The listing builds one solid part. Answer for the finished solid, in the listing's coordinates (mm). Round coordinates to 2 decimals unless told otherwise and drop trailing zeros. Loops run counter-clockwise (first coordinate to the right, second up) from the corner with the lowest first, then second, coordinate; pieces in that order, holes last. Notation, with made-up numbers: (-35, -36.5) -> (-28, -36.5) arc R23 ccw to (-28, 2.5) -> close; hole circle Ø4 at (28, -10). An arc over 180 degrees is marked (long way). One line per question, with ' | ' between items.
from build123d import *

# Parameters (mm, degrees)
SKETCH1_W           = 75
SKETCH1_H           = 60
BOSS_EXTRUDE1_DEPTH = 70
CAVITY1_START       = 5
CAVITY1_OUTLINE_R   = 0.75
CAVITY1_DEPTH       = 55.9
CAVITY1_2_OUTLINE_R = 0.75
CAVITY1_2_DEPTH     = 31.4
CAVITY1_START_2     = 13
CAVITY1_3_OUTLINE_R = 0.75
CAVITY1_3_DEPTH     = 47.9
CAVITY1_4_OUTLINE_R = 0.75
CAVITY1_4_DEPTH     = 23.4


# Read off the part's stored shape, not the designer's step: Cavity1
with BuildPart() as part:
    # Sketch1 → Boss-Extrude1 (new body)
    with BuildSketch(Plane.XY):
        with Locations((37.5, 30)):
            Rectangle(SKETCH1_W, SKETCH1_H)
    extrude(amount=BOSS_EXTRUDE1_DEPTH)

    # Cavity1 outline → Cavity1 (cut)
    with BuildSketch(Plane.XY.offset(CAVITY1_START)):
        with BuildLine():
            Line((18.46548662, 52.336946082), (7.908006381, 37.670492946))
            Line((7.908006381, 37.670492946), (9.936997433, 36.209946709))
            ThreePointArc((9.936997433, 36.209946709), (8.94403376, 33.444468797), (9.567109894, 30.572949848))
            Line((9.567109894, 30.572949848), (8.245641386, 29.863216812))
            Line((8.245641386, 29.863216812), (18.37116603, 11.010266096))
            Line((18.37116603, 11.010266096), (21.895082052, 12.902887525))
            Line((21.895082052, 12.902887525), (11.769557408, 31.755838241))
            ThreePointArc((11.769557408, 31.755838241), (11.438668953, 33.280776232), (11.965988485, 34.749400472))
            Line((11.965988485, 34.749400472), (20.056953769, 45.989370661))
            ThreePointArc((20.056953769, 45.989370661), (21.356620935, 46.794592998), (22.845349854, 46.446449406))
            ThreePointArc((22.845349854, 46.446449406), (23.927028985, 45.897391402), (25.123551575, 45.697821555))
            Line((25.123551575, 45.697821555), (50.502868756, 45.366563013))
            ThreePointArc((50.502868756, 45.366563013), (52.616494227, 45.804976964), (54.348334803, 47.093521742))
            ThreePointArc((54.348334803, 47.093521742), (56.461375235, 48.37027811), (58.92150101, 48.163329184))
            Line((58.92150101, 48.163329184), (58.956655303, 50.856669359))
            ThreePointArc((58.956655303, 50.856669359), (53.544792902, 53.606340424), (47.557302608, 54.60579307))
            Line((47.557302608, 54.60579307), (23.587024567, 54.918660406))
            ThreePointArc((23.587024567, 54.918660406), (20.710384856, 54.254419425), (18.46548662, 52.336946082))
        make_face()
        with Locations((18.756110409, 15.069070512)):
            Circle(CAVITY1_OUTLINE_R, mode=Mode.SUBTRACT)
        with Locations((37.538899797, 50.828307501)):
            Circle(CAVITY1_OUTLINE_R, mode=Mode.SUBTRACT)
    extrude(amount=CAVITY1_DEPTH, mode=Mode.SUBTRACT)

    # Cavity1 2 outline → Cavity1 2 (cut)
    # profile 1 of 2: a face of its own
    with BuildSketch(Plane.XY.offset(CAVITY1_START)):
        with BuildLine():
            Line((61.054335289, 50.521376908), (55.041269461, 53.046995369))
            ThreePointArc((55.041269461, 53.046995369), (57.060573485, 52.061967221), (58.956655303, 50.856669359))
            Line((58.956655303, 50.856669359), (58.92150101, 48.163329184))
            Line((58.92150101, 48.163329184), (59.892586686, 47.755452074))
            ThreePointArc((59.892586686, 47.755452074), (60.952620575, 47.155751273), (61.844382404, 46.326249172))
            Line((61.844382404, 46.326249172), (66.312422732, 41.068244262))
            ThreePointArc((66.312422732, 41.068244262), (66.987141001, 40.054307304), (67.407914577, 38.911388893))
            Line((67.407914577, 38.911388893), (69.018283104, 32.201939348))
            ThreePointArc((69.018283104, 32.201939348), (69.162099385, 30.992547032), (69.021092891, 29.782823896))
            Line((69.021092891, 29.782823896), (67.426314651, 23.069651593))
            ThreePointArc((67.426314651, 23.069651593), (67.008197192, 21.925758816), (66.335836102, 20.910257235))
            Line((66.335836102, 20.910257235), (61.88002209, 15.641887326))
            ThreePointArc((61.88002209, 15.641887326), (60.948767594, 14.725996436), (59.86612003, 13.995267134))
            Line((59.86612003, 13.995267134), (51.713665819, 9.520058721))
            ThreePointArc((51.713665819, 9.520058721), (46.306249088, 7.211864539), (40.551434527, 6.007694509))
            ThreePointArc((40.551434527, 6.007694509), (32.152585039, 5.712059517), (23.799153538, 6.633067087))
            Line((23.799153538, 6.633067087), (23.436550639, 4.666211949))
            ThreePointArc((23.436550639, 4.666211949), (32.077975822, 3.713451636), (40.766384828, 4.019278967))
            ThreePointArc((40.766384828, 4.019278967), (45.667164707, 4.941518532), (50.36406223, 6.617025293))
            Line((50.36406223, 6.617025293), (53.157281436, 6.890234782))
            Line((53.157281436, 6.890234782), (61.309735647, 11.365443195))
            ThreePointArc((61.309735647, 11.365443195), (62.847708644, 12.403492855), (64.170617702, 13.704576886))
            Line((64.170617702, 13.704576886), (68.626431714, 18.972946795))
            ThreePointArc((68.626431714, 18.972946795), (69.686109361, 20.573432518), (70.345085218, 22.37626975))
            Line((70.345085218, 22.37626975), (71.939863457, 29.089442053))
            ThreePointArc((71.939863457, 29.089442053), (72.162097362, 30.99603151), (71.93543508, 32.902099577))
            Line((71.93543508, 32.902099577), (70.325066554, 39.611549122))
            ThreePointArc((70.325066554, 39.611549122), (69.661904513, 41.4128507), (68.598511823, 43.010870491))
            Line((68.598511823, 43.010870491), (64.130471496, 48.268875401))
            ThreePointArc((64.130471496, 48.268875401), (62.725006351, 49.576215828), (61.054335289, 50.521376908))
        make_face()
        with Locations((55.111079675, 9.691018641)):
            Circle(CAVITY1_2_OUTLINE_R, mode=Mode.SUBTRACT)
    # profile 2 of 2: a face of its own
    with BuildSketch(Plane.XY.offset(CAVITY1_START)):
        with BuildLine():
            Line((21.895082052, 12.902887525), (20.133124041, 11.956576811))
            ThreePointArc((20.133124041, 11.956576811), (22.633217451, 9.122098941), (26.13158906, 7.691669655))
            ThreePointArc((26.13158906, 7.691669655), (41.165451618, 7.861619441), (55.287009069, 13.021805628))
            Line((55.287009069, 13.021805628), (54.29349955, 14.757587538))
            ThreePointArc((54.29349955, 14.757587538), (40.805776793, 9.829012137), (26.446697007, 9.66669041))
            ThreePointArc((26.446697007, 9.66669041), (23.79214447, 10.752095311), (21.895082052, 12.902887525))
        make_face()
    extrude(amount=CAVITY1_2_DEPTH, mode=Mode.SUBTRACT)

    # Cavity1 3 outline → Cavity1 3 (cut)
    with BuildSketch(Plane.XY.offset(CAVITY1_START_2)):
        with Locations((18.756110409, 15.069070512)):
            Circle(CAVITY1_3_OUTLINE_R)
        with Locations((37.538899797, 50.828307501)):
            Circle(CAVITY1_3_OUTLINE_R)
    extrude(amount=CAVITY1_3_DEPTH, mode=Mode.SUBTRACT)

    # Cavity1 4 outline → Cavity1 4 (cut)
    with BuildSketch(Plane.XY.offset(CAVITY1_START_2)):
        with Locations((55.111079675, 9.691018641)):
            Circle(CAVITY1_4_OUTLINE_R)
    extrude(amount=CAVITY1_4_DEPTH, mode=Mode.SUBTRACT)


solid = part.part
Q1. A cutting plane is placed at C-C on x = 34. Give the vertices of the cut face in (y, z), plus the area to 3 significant figures.
Numbers:
outline: (0, 0) -> (60, 0) -> (60, 70) -> (0, 70) -> close; hole (3.67, 5) -> (5.67, 5) -> (5.67, 36.4) -> (3.67, 36.4) -> close; hole (7.14, 5) -> (9.14, 5) -> (9.14, 36.4) -> (7.14, 36.4) -> close; hole (45.58, 5) -> (54.78, 5) -> (54.78, 60.9) -> (45.58, 60.9) -> close | area: 3,560 mm^2
Q2. A cutting plane is placed at D-D on y = 25. Give the vertices of the cut face in (x, z).
Numbers:
outline: (0, 0) -> (75, 0) -> (75, 70) -> (0, 70) -> close; hole (10.86, 5) -> (15.4, 5) -> (15.4, 60.9) -> (10.86, 60.9) -> close; hole (67.88, 5) -> (70.97, 5) -> (70.97, 36.4) -> (67.88, 36.4) -> close
Q3. A cutting plane is placed at B-B on y = 17. Give the vertices of the cut face in (x, z), plus the area to 3 significant figures.
Numbers:
outline: (0, 0) -> (75, 0) -> (75, 70) -> (0, 70) -> close; hole (15.15, 5) -> (19.69, 5) -> (19.69, 60.9) -> (15.15, 60.9) -> close; hole (63.03, 5) -> (66.96, 5) -> (66.96, 36.4) -> (63.03, 36.4) -> close | area: 4,870 mm^2
Q4. For a pull along Z with two mould halves and no side action, classify faces 1 (the face through (0, 30, 35)), 2 (the face through (69.674, 41.389, 20.48)), 3 (the face through (40.957, 7.824, 20.48)) as pulls with the +Z half, pulls with the -Z half, needs draft (parallel to the pull), parting line crosses it, or undercut.
Numbers:
face 1: needs draft | face 2: undercut | face 3: undercut
Q5. A cutting plane is placed at A-A on z = 46. Give the vertices of the cut face in (x, y).
Numbers:
outline: (0, 0) -> (75, 0) -> (75, 60) -> (0, 60) -> close; hole (7.91, 37.67) -> (9.94, 36.21) arc R5.33 ccw to (9.57, 30.57) -> (8.25, 29.86) -> (18.37, 11.01) -> (21.9, 12.9) -> (11.77, 31.76) arc R2.83 cw to (11.97, 34.75) -> (20.06, 45.99) arc R2 cw to (22.85, 46.45) arc R4 ccw to (25.12, 45.7) -> (50.5, 45.37) arc R5 ccw to (54.35, 47.09) arc R4 cw to (58.92, 48.16) -> (58.96, 50.86) arc R20 ccw to (47.56, 54.61) -> (23.59, 54.92) arc R6.21 ccw to (18.47, 52.34) -> close
Q6. Given pin 1 Ø10 at (y, z) = (20, 49) entering from -X, flat-ended and moving along its own axis, determine where the tip first touches the part or whether it passes through.
Numbers:
pin 1: x = 0
Q7. Find the intervals of material crossed by line 1 (Z direction, x = 22, y = 47.5); line 2 (X direction, y = 23, z = 19); line 3 (Y direction, x = 50.5, z = 45.5), in increasing order. Write a range as from..to.
Numbers:
line 1: 0..5, 60.9..70 | line 2: 0..11.93, 16.47..67.41, 70.49..75 | line 3: 0..45.37, 54.35..60
